Geometry check sheet. Reference: the model listing, model coordinates, mm. A direction names the side the tool comes from. Coordinates: 2 decimals unless noted, no trailing zeros. Order: outer loops, then holes, each group sorted by start corner. A loop starts at its lowest first (then second) coordinate and runs counter-clockwise, first axis right, second up. Notation, with made-up numbers: (-15, 54) - (10, 54) arc R26 cw to (10, 77) - close; hole circle Ø7 at (41, -13.5). An arc over 180 degrees is marked (long way). Return JSON: item names as keys, results as strings. Group by question number.
Item 1: Section check A-A on z = -2.5. Enter the section's corners in (x, y).
Item 2: Section check B-B on x = 2.25. Enter the section's corners in (y, z).
Item 3: Scan lines: probe 1 along X at (y, z) = (-0.4, -5.5); probe 2 along Z at (x, y) = (-0.25, -0.9); probe 3 along Z at (x, y) = (2, 0.35). Record each from-to range of solid material in increasing order.
Item 4: Draft check along X on faces 6 (the flat face through (7, 0, 15)), 7 (the flat face through (-9, 0, 0)), 8 (the flat face through (-1.55, 0, -3)). Enter one of: pulls with the +X half, pulls with the -X half, needs draft (parallel to the pull), parting line crosses it, or undercut.
Item 5: Gauge pin test, flat ends, axial feed: pin 1 (0.9 mm diameter, centred on x = 7.5, y = 0.5, fed in from +Z); pin 2 (0.9 mm diameter, centred on y = -0.5, z = 16, fed in from -X); pin 3 (0.5 mm diameter, centred on x = 0, y = -0.5, fed in from +Z). Record the tip position at first contact, or that the pin passes through.
Item 6: Section check D-D on x = -7. Enter the section's corners in (y, z), then the cut area to 3 significant figures.
Item 7: Section check C-C on y = 0.9. Enter the section's corners in (x, z), then the cut area to 3 significant figures.
Item 8: Tool access check on faces 1 (the flat face through (0, 0, -15)), 2 (the flat face through (2.85, 0, 13)), 3 (the flat face through (1.5, 0, 16)), 4 (the flat face through (6, 0, 17)), 5 (the flat face through (-6, 0, 17)). Record the directions out of +Z, -Z, +X, -X, +Y, -Y that give a thin tool (end or side, any length) a straight path to the whole face; none if there is none.
from build123d import *

# Parameters (mm, degrees)
SKETCH1_W               = 18
SKETCH1_H               = 30
BOSS_EXTRUDE1_DEPTH     = 1.5
SKETCH2_W               = 12
SKETCH2_H               = 3
BOSS_EXTRUDE2_DEPTH     = 1.5
CUT_EXTRUDE2_DEPTH      = 21.180436071
CUT_EXTRUDE2_DEPTH_BACK = 21.180436071
CUT_EXTRUDE1_DEPTH      = 21.180436071
CUT_EXTRUDE1_DEPTH_BACK = 21.180436071
SKETCH3_W               = 3.1
SKETCH3_H               = 6.6


with BuildPart() as part:
    # Sketch1 → Boss-Extrude1 (new, symmetric)
    with BuildSketch(Plane(origin=(0, 0, 0), x_dir=(1, 0, 0), z_dir=(0, 1, 0))):
        Rectangle(SKETCH1_W, SKETCH1_H)
    extrude(amount=BOSS_EXTRUDE1_DEPTH, both=True)

    # Sketch2 → Boss-Extrude2 (add, symmetric)
    with BuildSketch(Plane(origin=(0, 0, 0), x_dir=(1, 0, 0), z_dir=(0, 1, 0))):
        with Locations((0, -16.5)):
            Rectangle(SKETCH2_W, SKETCH2_H)
    extrude(amount=BOSS_EXTRUDE2_DEPTH, both=True)

    # Sketch4 → Cut-Extrude2 (cut, two sides: drawn at the far end of the back side and taken through both)
    with BuildSketch(Plane(origin=(0, 0, 0), x_dir=(1, 0, 0), z_dir=(0, 1, 0)).offset(-CUT_EXTRUDE2_DEPTH_BACK)):
        with BuildLine():
            Line((-1.5, -18), (1.5, -18))
            Line((1.5, -18), (1.5, -13.996114826))
            Line((1.5, -13.996114826), (2.85, -13.996114826))
            Line((2.85, -13.996114826), (2.85, -11.726114826))
            Line((2.85, -11.726114826), (1.5, -11.726114826))
            Line((1.5, -11.726114826), (1.5, -9))
            ThreePointArc((1.5, -9), (1.207106781, -8.292893219), (0.5, -8))
            Line((0.5, -8), (-0.5, -8))
            ThreePointArc((-0.5, -8), (-1.207106781, -8.292893219), (-1.5, -9))
            Line((-1.5, -9), (-1.5, -11.726114826))
            Line((-1.5, -11.726114826), (-2.85, -11.726114826))
            Line((-2.85, -11.726114826), (-2.85, -13.996114826))
            Line((-2.85, -13.996114826), (-1.5, -13.996114826))
            Line((-1.5, -13.996114826), (-1.5, -18))
        make_face()
    extrude(amount=CUT_EXTRUDE2_DEPTH + CUT_EXTRUDE2_DEPTH_BACK, mode=Mode.SUBTRACT)

    # Sketch3 → Cut-Extrude1 (cut, two sides: drawn at the far end of the back side and taken through both)
    with BuildSketch(Plane(origin=(0, 0, 0), x_dir=(1, 0, 0), z_dir=(0, 1, 0)).offset(-CUT_EXTRUDE1_DEPTH_BACK)):
        with Locations((0, 3)):
            Rectangle(SKETCH3_W, SKETCH3_H)
    extrude(amount=CUT_EXTRUDE1_DEPTH + CUT_EXTRUDE1_DEPTH_BACK, mode=Mode.SUBTRACT)


solid = part.part
Computed:
{
 "1": {"outline": "(-9, -1.5) - (-1.55, -1.5) - (-1.55, 1.5) - (-9, 1.5) - close; (1.55, -1.5) - (9, -1.5) - (9, 1.5) - (1.55, 1.5) - close"},
 "2": {"outline": "(-1.5, -15) - (1.5, -15) - (1.5, 11.73) - (-1.5, 11.73) - close; (-1.5, 14) - (1.5, 14) - (1.5, 18) - (-1.5, 18) - close"},
 "3": {"probe 1": "x = -9 to -1.55, 1.55 to 9", "probe 2": "z = -15 to -6.3, 0.3 to 8", "probe 3": "z = -15 to 11.73, 14 to 18"},
 "4": {"face 6": "needs draft", "face 7": "pulls with the -X half", "face 8": "undercut"},
 "5": {"pin 1": "stops at z = 15", "pin 2": "stops at x = -6", "pin 3": "stops at z = 8"},
 "6": {"outline": "(-1.5, -15) - (1.5, -15) - (1.5, 15) - (-1.5, 15) - close", "area": "90.0 mm²"},
 "7": {"outline": "(-9, -15) - (9, -15) - (9, 15) - (6, 15) - (6, 18) - (1.5, 18) - (1.5, 14) - (2.85, 14) - (2.85, 11.73) - (1.5, 11.73) - (1.5, 9) arc R1 cw to (0.5, 8) - (-0.5, 8) arc R1 cw to (-1.5, 9) - (-1.5, 11.73) - (-2.85, 11.73) - (-2.85, 14) - (-1.5, 14) - (-1.5, 18) - (-6, 18) - (-6, 15) - (-9, 15) - close; hole (-1.55, -6.3) - (1.55, -6.3) - (1.55, 0.3) - (-1.55, 0.3) - close", "area": "520 mm²"},
 "8": {"face 1": "-Z, +X, -X, +Y, -Y", "face 2": "+Y, -Y", "face 3": "+Z, +Y, -Y", "face 4": "+Z, +X, +Y, -Y", "face 5": "+Z, -X, +Y, -Y"}
}
